```python
from build123d import *

# Parameters (mm, degrees)
F1_DEPTH = 38.1
F2_W     = 19.05
F2_H     = 69.85
F3_DEPTH = 19.05


# Not quite as in the source:
# - a pattern or mirror of a feature is missing from the dataset's text; its kind, count and spacing are read off the source's solid


with BuildPart() as f1:
    # F0 (on Front) → F1 (new body)
    with BuildSketch(Plane.XZ):
        with BuildLine():
            ThreePointArc((25.4, 147.32), (495.3, 299.72), (965.2, 147.32))
            Line((965.2, 147.32), (965.2, 246.8872163374))
            ThreePointArc((965.2, 246.8872163374), (790.2509366907, 331.5626859382), (601.016852567, 375.92))
            Line((601.016852567, 375.92), (389.583147433, 375.92))
            ThreePointArc((389.583147433, 375.92), (200.3490633093, 331.5626859382), (25.4, 246.8872163374))
            Line((25.4, 246.8872163374), (25.4, 217.17))
            Line((25.4, 217.17), (25.4, 153.67))
            Line((25.4, 153.67), (25.4, 147.32))
        make_face()
    extrude(amount=F1_DEPTH)

    # F2 (on face) → F3 (join)
    with BuildSketch(Plane.YZ.offset(965.2)):
        with Locations((-19.05, 188.595)):
            Rectangle(F2_W, F2_H)
    f3 = extrude(amount=F3_DEPTH)

    # F3_copies: F3 across plane
    add(f3.mirror(Plane(origin=(495.3, 0, 0), x_dir=(0, 0, -1), z_dir=(-1, 0, 0))))


solid = f1.part
```
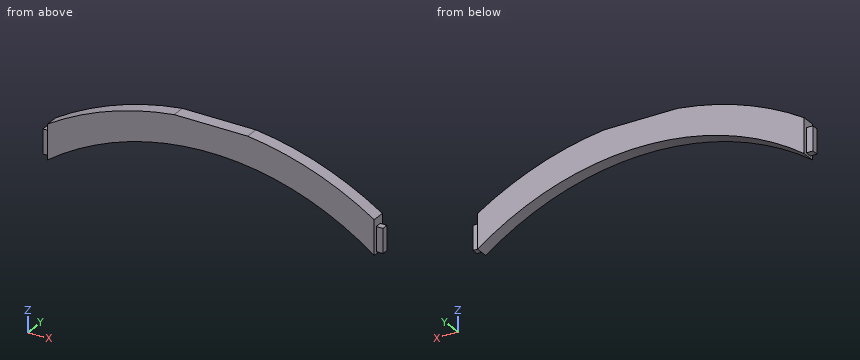
Can you work these out from the model? Positions are in its coordinate system, mm. Round coordinates to 2 decimals unless told otherwise and drop trailing zeros. Loops run counter-clockwise (first coordinate to the right, second up) from the corner with the lowest first, then second, coordinate; pieces in that order, holes last. Notation, with made-up numbers: (11.25, 53.25) -> (25.25, 53.25) arc R27 ccw to (25.25, 78.25) -> close; hole circle Ø11 at (88.25, 40.5). An arc over 180 degrees is marked (long way). Answer in a Markdown table with one row per item.
Item 1: Suppose I cut it at C-C, the plane z = 174.5. List the corners of the cut face in (x, y) for me (3 decimals), plus the area to 3 significant figures.
Answer block:
| item | result |
|---|---|
| outline | (6.35, -28.575) -> (25.4, -28.575) -> (25.4, -38.1) -> (65.382, -38.1) -> (65.382, 0) -> (25.4, 0) -> (25.4, -9.525) -> (6.35, -9.525) -> close; (925.218, -38.1) -> (965.2, -38.1) -> (965.2, -28.575) -> (984.25, -28.575) -> (984.25, -9.525) -> (965.2, -9.525) -> (965.2, 0) -> (925.218, 0) -> close |
| area | 3,770 mm² |
Item 2: If I drill on probe 1 along X at (y, z) = (-23.5, 180); probe 2 along Z at (x, y) = (637.5, -27); probe 3 along X at (y, z) = (-16, 185), over which ranges is the centre line in solid material (lowest first)?
Answer block:
| item | result |
|---|---|
| probe 1 | 6.35 to 74.15, 916.45 to 984.25 |
| probe 2 | 286.99 to 370.75 |
| probe 3 | 6.35 to 82.34, 908.26 to 984.25 |
Item 3: Suppose I cut it at D-D, the plane x = 265.5. List the corners of the cut face in (y, z) for me, plus the area to 3 significant figures.
Answer block:
| item | result |
|---|---|
| outline | (-38.1, 266.03) -> (0, 266.03) -> (0, 351.85) -> (-38.1, 351.85) -> close |
| area | 3,270 mm² |
Item 4: Will these pins go through, and if not, where does the flat tip stop? P1, Ø21, axis at x = 976.5, y = -18.5, coming from the -Z side; P2, Ø9.5, axis at x = 974, y = -19.5, coming from the +Z side; P3, Ø21, axis at x = 20, y = -14.5, coming from the +Z side.
Answer block:
| item | result |
|---|---|
| P1 | z = 153.67 |
| P2 | z = 223.52 |
| P3 | z = 250.07 |
Item 5: Suppose I cut it at A-A, the plane z = 234.5. List the corners of the cut face in (x, y) for me, plus the area to 3 significant figures.
Answer block:
| item | result |
|---|---|
| outline | (25.4, -38.1) -> (178.79, -38.1) -> (178.79, 0) -> (25.4, 0) -> close; (811.81, -38.1) -> (965.2, -38.1) -> (965.2, 0) -> (811.81, 0) -> close |
| area | 11,700 mm² |
Item 6: Suppose I cut it at B-B, the plane y = -20. List the corners of the cut face in (x, z) for me.
Answer block:
| item | result |
|---|---|
| outline | (6.35, 153.67) -> (25.4, 153.67) -> (25.4, 147.32) arc R800.63 cw to (965.2, 147.32) -> (965.2, 153.67) -> (984.25, 153.67) -> (984.25, 223.52) -> (965.2, 223.52) -> (965.2, 246.89) arc R883.18 ccw to (601.02, 375.92) -> (389.58, 375.92) arc R883.18 ccw to (25.4, 246.89) -> (25.4, 223.52) -> (6.35, 223.52) -> close |
